Here's how the part is built. I have some questions about the finished solid (model axes, mm). Give positions to 0.01 mm unless a question says otherwise; leave off trailing zeros. Order: outer loops, then holes, each group sorted by start corner. A loop starts at its lowest first (then second) coordinate and runs counter-clockwise, first axis right, second up.
from build123d import *

# Parameters (mm, degrees)
F1_DEPTH    = 3.9878
F2_T1_DEPTH = 229.3282991577
F2_T3_DEPTH = 66.1332991577


# Not quite as in the source:
# - a fillet or chamfer that OpenCascade refuses, or shapes differently, is made with other operations: its cross-section is extruded or revolved along the edge and cut away or added


with BuildPart() as f1:
    # F0 (on Front) → F1 (new body)
    with BuildSketch(Plane.XZ):
        with BuildLine():
            Line((0, -20.0025), (101.6, -20.0025))
            Line((101.6, -20.0025), (101.6, 0))
            Line((101.6, 0), (87.21852, 0))
            ThreePointArc((87.21852, 0), (83.82, -3.39852), (80.42148, 0))
            Line((80.42148, 0), (44.0436, 0))
            ThreePointArc((44.0436, 0), (40.64, -3.4036), (37.2364, 0))
            Line((37.2364, 0), (0, 0))
            Line((0, 0), (0, -20.0025))
        make_face()
        Polygon((-101.6, -20.0025), (0, -20.0025), (0, 0), (0, 20.0025), (-101.6, 20.0025), (-101.6, 0), align=None)
        with BuildLine():
            ThreePointArc((-72.80148, 0), (-76.2, -3.39852), (-79.59852, 0))
            ThreePointArc((-79.59852, 0), (-76.2, 3.39852), (-72.80148, 0))
        make_face(mode=Mode.SUBTRACT)
        with BuildLine():
            Line((87.21852, 0), (101.6, 0))
            Line((101.6, 0), (101.6, 20.0025))
            Line((101.6, 20.0025), (0, 20.0025))
            Line((0, 20.0025), (0, 0))
            Line((0, 0), (37.2364, 0))
            ThreePointArc((37.2364, 0), (40.64, 3.4036), (44.0436, 0))
            Line((44.0436, 0), (80.42148, 0))
            ThreePointArc((80.42148, 0), (83.82, 3.39852), (87.21852, 0))
        make_face()
    extrude(amount=F1_DEPTH)

    # F2: chamfer of 5.08 on 4 edges, made by hand

    # F2_s2 → F2_t1 (cut)
    with BuildSketch(Plane.YZ.offset(-114.6641495789)):
        Polygon((1.0922, 20.0025), (-3.9878, 14.9225), (-3.9878, 20.0025), align=None)
        Polygon((1.0922, -20.0025), (-3.9878, -14.9225), (-3.9878, -20.0025), align=None)
    extrude(amount=F2_T1_DEPTH, mode=Mode.SUBTRACT)

    # F2_s4 → F2_t3 (cut)
    with BuildSketch(Plane.XY.offset(-33.0666495789)):
        Polygon((-101.6, 1.0922), (-96.52, -3.9878), (-101.6, -3.9878), align=None)
        Polygon((101.6, 1.0922), (96.52, -3.9878), (101.6, -3.9878), align=None)
    extrude(amount=F2_T3_DEPTH, mode=Mode.SUBTRACT)


solid = f1.part
Q1. If we section it at A-A on x = -76.2: List the corners of the cut face in (y, z) for me.
Filled sheet:
outline: (-3.99, -14.92) - (0, -18.91) - (0, -3.4) - (-3.99, -3.4) - close; (-3.99, 3.4) - (0, 3.4) - (0, 18.91) - (-3.99, 14.92) - close
Q2. Thinking about a two-plate mould opening in X: for faces 1 (the face through (98.54, -1.97, -0.26)), 2 (the face through (-72.805, -1.966, 0.149)), 3 (the face through (-1, 0, 0)), which applies, released by +X, released by -X, zero draft, split by the parting line, or undercut?
Filled sheet:
face 1: released by +X
face 2: undercut
face 3: zero draft
Q3. If we section it at C-C on y = -0.7: List the corners of the cut face in (x, z) for me.
Filled sheet:
outline: (-99.81, -18.21) - (99.81, -18.21) - (99.81, 18.21) - (-99.81, 18.21) - close; hole circle Ø6.8 at (-76.2, 0); hole circle Ø6.81 at (40.64, 0); hole circle Ø6.8 at (83.82, 0)
Q4. If we section it at B-B on z = 0: List the corners of the cut face in (x, y) for me, plus the area to 3 significant figures.
Filled sheet:
outline: (-100.51, 0) - (-96.52, -3.99) - (-79.6, -3.99) - (-79.6, 0) - close; (-72.8, -3.99) - (37.24, -3.99) - (37.24, 0) - (-72.8, 0) - close; (44.04, -3.99) - (80.42, -3.99) - (80.42, 0) - (44.04, 0) - close; (87.22, -3.99) - (96.52, -3.99) - (100.51, 0) - (87.22, 0) - close
area: 704 mm2
Q5. I need wall thicknesses on L1, parallel to X at y = -3.7, z = -1; L2, parallel to Z at x = 83.82, y = -0.9; L3, parallel to Z at x = -76.2, y = -3. Which ranges of each line are inside material? Lowest first, please.
Filled sheet:
L1: x = -96.81 to -79.45, -72.95 to 37.39, 43.89 to 80.57, 87.07 to 96.81
L2: z = -18.01 to -3.4, 3.4 to 18.01
L3: z = -15.91 to -3.4, 3.4 to 15.91
Q6. I'm going to push a flat-ended pin straight in: P1, Ø1, axis at x = -45.5, y = -1.5, coming from the -Z side. Where does the tip first touch, or does it pass through?
Filled sheet:
P1: stops at z = -17.91
